```python
from build123d import *

# Parameters (mm, degrees)
F3_DEPTH = 12.5
F5_DEPTH = 12.5
F6_SIZE  = 0.1


with BuildPart() as f1:
    # F0 (on Front) → F1 (revolve)
    with BuildSketch(Plane.XZ):
        with BuildLine():
            Line((-30, 1.25), (-30, 0))
            Line((-30, 0), (28.4, 0))
            Line((28.4, 0), (28.4, 2))
            Line((28.4, 2), (18.23303, 2))
            ThreePointArc((18.23303, 2), (17.316515, 1.4), (16.4, 2))
            Line((16.4, 2), (-10.6, 2))
            Line((-10.6, 2), (-10.6, 3.35))
            Line((-10.6, 3.35), (-21.5, 3.35))
            Line((-21.5, 3.35), (-21.5, 1.25))
            Line((-21.5, 1.25), (-30, 1.25))
        make_face()
    revolve(axis=Axis((0, 0, 0), (1, 0, 0)))

    # F2 (on Top) → F3 (cut, symmetric)
    with BuildSketch(Plane.XY):
        Polygon((28.4, -2), (28.4, 0), (23.4, 0), (22.750161, -2), align=None)
    extrude(amount=F3_DEPTH, both=True, mode=Mode.SUBTRACT)

    # F4 (on Top) → F5 (cut, symmetric)
    with BuildSketch(Plane.XY):
        Polygon((-30, 1.25), (-30, 0.225), (-28.2, 1.25), align=None)
        Polygon((-28.2, -1.25), (-30, -0.225), (-30, -1.25), align=None)
    extrude(amount=F5_DEPTH, both=True, mode=Mode.SUBTRACT)

    # F6
    f6_edges = [f1.edges().sort_by_distance(p)[0] for p in [
        (-10.6, 0, -3.35),
        (-21.5, 0, -3.35),
    ]]
    chamfer(f6_edges, length=F6_SIZE)


solid = f1.part
```
Source: CAD feature listing. Evaluate the final solid. Frame: model axes, mm. A direction names the side the tool comes from. Round coordinates to 2 decimals unless told otherwise and drop trailing zeros. Loops run counter-clockwise (first coordinate to the right, second up) from the corner with the lowest first, then second, coordinate; pieces in that order, holes last.
(1) Access query for faces 1 (the cylindrical face through (-24.865, -0.845, -0.921)), 2 (the flat face through (-29.31, 0.62, -0.02)), 3 (the flat face through (-10.6, 2, -1)), 4 (the flat face through (26, 0, 0)), 5 (the flat face through (28.4, 1, 0)). Directions: +Z, -Z, +X, -X, +Y, -Y. A direction counts if a zero-diameter tool reaches every point of the face in a straight line with its end or side. Return the directions, or none.
From the geometry:
face 1: -X
face 2: +Z, -Z, -X, +Y
face 3: +X
face 4: +Z, -Z, +X, -Y
face 5: +Z, -Z, +X, +Y, -Y
(2) Section query B-B (x = 8). Output: boundary loops of the cut face in (y, z).
From the geometry:
outline: circle Ø4 at (0, 0)
(3) Section query A-A (z = 0). Output: boundary loops of the cut face in (x, y) (3 decimals), and give its area (3 significant figures).
From the geometry:
outline: (-30, -0.225) - (-28.2, -1.25) - (-21.5, -1.25) - (-21.5, -3.25) - (-21.4, -3.35) - (-10.7, -3.35) - (-10.6, -3.25) - (-10.6, -2) - (16.4, -2) arc R1 cw to (18.233, -2) - (22.75, -2) - (23.4, 0) - (28.4, 0) - (28.4, 2) - (18.233, 2) arc R1 cw to (16.4, 2) - (-10.6, 2) - (-10.6, 3.25) - (-10.7, 3.35) - (-21.4, 3.35) - (-21.5, 3.25) - (-21.5, 1.25) - (-28.2, 1.25) - (-30, 0.225) - close
area: 236 mm2
(4) Section query D-D (x = 24.5). Output: boundary loops of the cut face in (y, z).
From the geometry:
outline: (0, -2) arc R2 ccw to (0, 2) - close
(5) Contact query for flat-ended pins moving along their axis: pin 1 Ø2 at (x, z) = (26, 0.5) entering from -Y; pin 2 Ø1 at (x, z) = (-1.5, -1.5) entering from -Y; pin 3 Ø1.5 at (x, y) = (-1, -1.5) entering from +Z. Output: stop coordinate, or through.
From the geometry:
pin 1: stops at y = 0
pin 2: stops at y = -1.73
pin 3: stops at z = 1.85
(6) Section query C-C (x = -17.5). Output: boundary loops of the cut face in (y, z), and give its area (3 significant figures).
From the geometry:
outline: circle Ø6.7 at (0, 0)
area: 35.3 mm2
(7) Material intervals for probe 1 along X at (y, z) = (-1.5, -2); probe 2 along Y at (x, z) = (-1, 0); probe 3 along X at (y, z) = (-1.5, -0.5), sorted ascending.
From the geometry:
probe 1: x = -21.5 to -10.6
probe 2: y = -2 to 2
probe 3: x = -21.5 to 16.74, 17.89 to 22.91
